Read the model definition and answer for the solid it produces. Units are mm, in the model's axes. Face numbers are marked on the shaded views. A direction names the side the tool comes from. Round coordinates to 2 decimals unless told otherwise and drop trailing zeros. Order: outer loops, then holes, each group sorted by start corner. A loop starts at its lowest first (then second) coordinate and runs counter-clockwise, first axis right, second up. Notation, with made-up numbers: (44, -22.75) - (103, -22.75) arc R26 cw to (103, -3.75) - close; hole circle Ø7 at (46, 28). An arc over 180 degrees is marked (long way). Put each result on its own line as item: value. Start each with the question number.
Q1. Section D-D on z = 4 is taken. Give the vertices of the cut face in (x, y) (3 decimals), then the cut area to 3 significant figures.
Q2. Section A-A on x = 47 is taken. Give the vertices of the cut face in (y, z).
Q3. For a pull along Z with two mould halves and no side action, classify the marked faces 5, 6, 7 and 8 as pulls with the +Z half, pulls with the -Z half, needs draft (parallel to the pull), parting line crosses it, or undercut.
Q4. Section B-B on z = 11.5 is taken. Give the vertices of the cut face in (x, y).
Q5. Section C-C on y = 0 is taken. Give the vertices of the cut face in (x, z).
Q6. Each of these flat-tipped pins is pushed along its axis until it touches: pin 1 Ø1 at (y, z) = (-11, -12) entering from -X; pin 2 Ø1.6 at (y, z) = (-4.5, 10) entering from +X; pin 3 Ø2 at (x, z) = (3.5, 9.5) entering from +Y; pin 4 Ø3 at (x, y) = (13.5, 6.5) entering from -Z. Where does it stop, or does it pass through?
Q7. Which of the six approach directions +Z, -Z, +X, -X, +Y, -Y give full straight-line access (tool end or side, diameter ignored) to the marked faces 1, 2, 3 and 4?
Q8. Find the intervals of material crossed by line 1 along Z through (x, y) = (15.5, -2.25); line 2 along Z through (x, y) = (7, -6.75); line 3 along Y through (x, z) = (39, 0.75), in increasing order. Write a range as from..to.
from build123d import *

# Parameters (mm, degrees)
EXTRUDE1_DEPTH             = 12.954
SKETCH3_R                  = 5
CUT_EXTRUDE1_DEPTH         = 2.6162
CUT_EXTRUDE2_DEPTH         = 7.493
EXTRUDE2_REACH             = 14.954
EXTRUDE2_DIRECTION_2_REACH = 14.954
SKETCH7_W                  = 13.462
SKETCH7_H                  = 3.9878
CUT_EXTRUDE3_DEPTH         = 6.9944
CUT_EXTRUDE4_DEPTH         = 3.9972


with BuildPart() as part:
    # Sketch2 → Extrude1 (new body, symmetric)
    with BuildSketch(Plane.XY):
        with BuildLine():
            Line((37.9984, -11.5062), (37.9984, -1.4986))
            Line((37.9984, -1.4986), (11.036020087, 3.255595043))
            ThreePointArc((11.036020087, 3.255595043), (-9.215534877, 6.889597621), (0, -11.5062))
            Line((0, -11.5062), (37.9984, -11.5062))
        make_face()
    extrude(amount=EXTRUDE1_DEPTH, both=True)

    # Sketch3 → Cut-Extrude1 (cut)
    with BuildSketch(Plane.XY.offset(12.954)):
        with BuildLine():
            Line((0, -11.5062), (4.495154191, -11.5062))
            Line((4.495154191, -11.5062), (4.495154191, -10.5918))
            ThreePointArc((4.495154191, -10.5918), (-2.293607342, 11.27528287), (0, -11.5062))
        make_face()
        Circle(SKETCH3_R, mode=Mode.SUBTRACT)
    cut_extrude1 = extrude(amount=-CUT_EXTRUDE1_DEPTH, mode=Mode.SUBTRACT)

    # Mirror1: Cut-Extrude1 across plane
    add(cut_extrude1.mirror(Plane.XY), mode=Mode.SUBTRACT)

    # Sketch4 → Cut-Extrude2 (cut, symmetric)
    with BuildSketch(Plane.XY):
        with BuildLine():
            Line((8.9916, -8.509), (37.9984, -8.509))
            Line((37.9984, -8.509), (37.9984, -1.4986))
            Line((37.9984, -1.4986), (11.036020087, 3.255595043))
            ThreePointArc((11.036020087, 3.255595043), (-9.215534877, 6.889597621), (0, -11.5062))
            Line((0, -11.5062), (8.9916, -11.5062))
            Line((8.9916, -11.5062), (8.9916, -8.509))
        make_face()
    extrude(amount=CUT_EXTRUDE2_DEPTH, both=True, mode=Mode.SUBTRACT)

    # Extrude2: up to this face of the body (flat: up to its plane)
    extrude2_end = Plane(part.part.faces().sort_by_distance((8.815484891, -1.610467544, -7.493))[0])
    # Sketch5 → Extrude2 (add, up to the picked face)
    with BuildSketch(Plane.XY, mode=Mode.PRIVATE) as extrude2_sk1:
        Polygon((54.991, -5.5118), (38.0238, -5.5118), (38.0238, -8.509), (37.9984, -8.509), (37.9984, -11.5062), (40.005, -11.5062), (40.005, -9.4996), (54.991, -9.4996), align=None)
    extrude2_tool1 = split(extrude(extrude2_sk1.sketch, amount=-EXTRUDE2_REACH, mode=Mode.PRIVATE), bisect_by=extrude2_end, keep=Keep.BOTH, mode=Mode.PRIVATE)
    add(extrude2_tool1.solids().sort_by_distance((46.083002, -7.674508, 0))[0])

    # Extrude2 direction 2: up to this face of the body (flat: up to its plane)
    extrude2_direction_2_end = Plane(part.part.faces().sort_by_distance((8.815484891, -1.610467544, 7.493))[0])
    # Sketch5 → Extrude2 direction 2 (add, up to the picked face)
    with BuildSketch(Plane.XY, mode=Mode.PRIVATE) as extrude2_direction_2_sk1:
        Polygon((54.991, -5.5118), (38.0238, -5.5118), (38.0238, -8.509), (37.9984, -8.509), (37.9984, -11.5062), (40.005, -11.5062), (40.005, -9.4996), (54.991, -9.4996), align=None)
    extrude2_direction_2_tool1 = split(extrude(extrude2_direction_2_sk1.sketch, amount=EXTRUDE2_DIRECTION_2_REACH, mode=Mode.PRIVATE), bisect_by=extrude2_direction_2_end, keep=Keep.BOTH, mode=Mode.PRIVATE)
    add(extrude2_direction_2_tool1.solids().sort_by_distance((46.083002, -7.674508, 0))[0])

    # Sketch7 → Cut-Extrude3 (cut, through all)
    with BuildSketch(Plane(origin=(0, -5.5118, 0), x_dir=(1, 0, 0), z_dir=(0, 1, 0))):
        with Locations((48.26, 0)):
            Rectangle(SKETCH7_W, SKETCH7_H)
    extrude(amount=-CUT_EXTRUDE3_DEPTH, mode=Mode.SUBTRACT)

    # Sketch8 → Cut-Extrude4 (cut, through all)
    with BuildSketch(Plane(origin=(0, -8.509, 0), x_dir=(1, 0, 0), z_dir=(0, 1, 0))):
        with BuildLine():
            Line((19.7612, 2.2479), (19.7612, -2.2479))
            ThreePointArc((19.7612, -2.2479), (16.51, -5.4991), (13.2588, -2.2479))
            Line((13.2588, -2.2479), (13.2588, 2.2479))
            ThreePointArc((13.2588, 2.2479), (16.51, 5.4991), (19.7612, 2.2479))
        make_face()
        with BuildLine():
            Line((33.7566, 2.2479), (33.7566, -2.2479))
            ThreePointArc((33.7566, -2.2479), (30.5054, -5.4991), (27.2542, -2.2479))
            Line((27.2542, -2.2479), (27.2542, 2.2479))
            ThreePointArc((27.2542, 2.2479), (30.5054, 5.4991), (33.7566, 2.2479))
        make_face()
    extrude(amount=-CUT_EXTRUDE4_DEPTH, mode=Mode.SUBTRACT)


solid = part.part
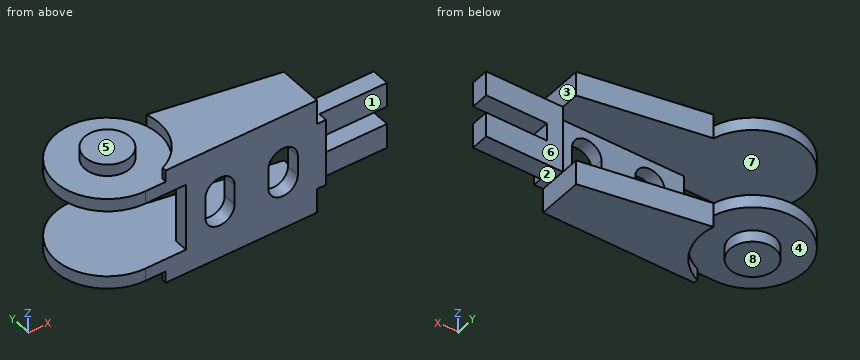
Findings:
1. outline: (8.992, -11.506) - (13.771, -11.506) - (13.771, -8.509) - (8.992, -8.509) - close; (19.249, -11.506) - (27.767, -11.506) - (27.767, -8.509) - (19.249, -8.509) - close; (33.244, -11.506) - (40.005, -11.506) - (40.005, -9.5) - (54.991, -9.5) - (54.991, -5.512) - (38.024, -5.512) - (38.024, -8.509) - (33.244, -8.509) - close
1. area: 126 mm2
2. outline: (-9.5, -7.49) - (-5.51, -7.49) - (-5.51, -1.99) - (-9.5, -1.99) - close; (-9.5, 1.99) - (-5.51, 1.99) - (-5.51, 7.49) - (-9.5, 7.49) - close
3. face 5: pulls with the +Z half
3. face 6: needs draft
3. face 7: undercut
3. face 8: pulls with the -Z half
4. outline: circle Ø10 at (0, 0); (4.5, -11.51) - (38, -11.51) - (38, -1.5) - (11.04, 3.26) arc R11.51 cw to (4.5, -10.59) - close
5. outline: (-11.51, -10.34) - (-5, -10.34) - (-5, -12.95) - (5, -12.95) - (5, -10.34) - (11.51, -10.34) - (11.51, -12.95) - (29.5, -12.95) - (29.5, -7.49) - (-11.51, -7.49) - close; (-11.51, 7.49) - (29.5, 7.49) - (29.5, 12.95) - (11.51, 12.95) - (11.51, 10.34) - (5, 10.34) - (5, 12.95) - (-5, 12.95) - (-5, 10.34) - (-11.51, 10.34) - close
6. pin 1: x = 4.5
6. pin 2: x = 38
6. pin 3: y = 11.23
6. pin 4: through
7. face 1: +Z, -Z, +X, -Y
7. face 2: -Z, +X, +Y, -Y
7. face 3: +Z, +X, +Y, -Y
7. face 4: -Z
8. line 1: -12.95..-7.49, 7.49..12.95
8. line 2: -10.34..-7.49, 7.49..10.34
8. line 3: -11.51..-5.51
